Geometry check sheet. Reference: the model listing, model coordinates, mm. A direction names the side the tool comes from. Give positions to 0.01 mm unless a question says otherwise; leave off trailing zeros. Loops run counter-clockwise (first coordinate to the right, second up) from the corner with the lowest first, then second, coordinate; pieces in that order, holes last. Notation, with made-up numbers: (18, -22) - (36, -22) arc R18 cw to (36, 9) - close; hole circle Ø5 at (24, 71.25). An arc over 180 degrees is marked (long way). Use a Markdown table: item, result. Add a question column.
1. Draft check along Y on faces 1 (the flat face through (-28.228, 1.807, 9.481)), 2 (the flat face through (-57.807, 6.439, 5.009)), 3 (the flat face through (-25, 1, 0)), 4 (the flat face through (-21.915, -29.438, 11.448)). Enter one of: pulls with the +Y half, pulls with the -Y half, needs draft (parallel to the pull), parting line crosses it, or undercut.
2. Cross-section at C-C on y = 13.5. Enter the section's corners in (x, z), and give its area (3 significant figures).
3. Cross-section at B-B on x = -10. Enter the section's corners in (y, z), and give its area (3 significant figures).
4. Material ranges on L1, parallel to Y at x = -6, z = 6.5; L2, parallel to Y at x = -36, z = 8; L3, parallel to Y at x = -45, z = 7, recorded low to high.
5. Set-up check for faces 5 (the flat face through (-44.25, 18.21, 11.41)), 6 (the flat face through (-21.97, -16.81, 9.57)): record each of +Z, -Z, +X, -X, +Y, -Y from which the full face is reachable in a straight line by a thin tool's end or side.
6. Cross-section at D-D on x = -27. Enter the section's corners in (y, z).
7. Cross-section at A-A on z = 4. Enter the section's corners in (x, y).
8. Depth check by flat-ended pin: P1, Ø5, axis at x = -28, z = 5, coming from the +Y side; P2, Ø5, axis at y = -16, z = 8, coming from the +X side; P3, Ø1.9, axis at y = 14, z = 9.5, coming from the +X side. Enter the tip coordinate at first touch or a pass-through.
from build123d import *

# Parameters (mm, degrees)
F1_DEPTH    = 12.7
F3_DEPTH    = 40.64
F4_DEPTH    = 53.34
F5_T1_DEPTH = 85.1725092407
F5_T3_DEPTH = 73.3110318687
F5_T5_DEPTH = 73.3110318687
F5_T7_DEPTH = 85.1725092407
F6_SIZE     = 2.54


# Not quite as in the source:
# - a fillet or chamfer that OpenCascade refuses, or shapes differently, is made with other operations: its cross-section is extruded or revolved along the edge and cut away or added


with BuildPart() as f1:
    # F0 (on Top) → F1 (new body)
    with BuildSketch(Plane.XY):
        Polygon((0, -38.1), (0, 38.1), (-38.1, 25.4), (-52.2708785332, 12.7), (-63.5, 0), (-52.2708785332, -12.7), (-38.1, -25.4), align=None)
    extrude(amount=F1_DEPTH)

    # F2 (on face) → F3 (cut)
    with BuildSketch(Plane.YZ):
        Polygon((-14.9523484187, 6.35), (-11.2861742094, 12.7), (-18.6185226281, 12.7), align=None)
        Polygon((18.6185226281, 12.7), (11.2861742094, 12.7), (14.9523484187, 6.35), align=None)
    extrude(amount=-F3_DEPTH, mode=Mode.SUBTRACT)

    # F2 (on face) → F4 (cut)
    with BuildSketch(Plane.YZ):
        Polygon((3.6661742094, 12.7), (-3.6661742094, 12.7), (0, 6.35), align=None)
    extrude(amount=-F4_DEPTH, mode=Mode.SUBTRACT)

    # F5: chamfer of 7.62 x 12.7 on 4 edges, made by hand

    # F5_s2 → F5_t1 (cut)
    with BuildSketch(Plane.XZ.offset(-14.2269933063)):
        Polygon((-7.62, 12.7), (0, 0), (0, 12.7), align=None)
    extrude(amount=F5_T1_DEPTH, mode=Mode.SUBTRACT)

    # F5_s4 → F5_t3 (cut)
    with BuildSketch(Plane.XZ.offset(-29.179341725)):
        Polygon((-7.62, 12.7), (0, 0), (0, 12.7), align=None)
    extrude(amount=F5_T3_DEPTH, mode=Mode.SUBTRACT)

    # F5_s6 → F5_t5 (cut)
    with BuildSketch(Plane.XZ.offset(-44.1316901437)):
        Polygon((-7.62, 12.7), (0, 0), (0, 12.7), align=None)
    extrude(amount=F5_T5_DEPTH, mode=Mode.SUBTRACT)

    # F5_s8 → F5_t7 (cut)
    with BuildSketch(Plane.XZ.offset(-70.9455159344)):
        Polygon((-7.62, 12.7), (0, 0), (0, 12.7), align=None)
    extrude(amount=F5_T7_DEPTH, mode=Mode.SUBTRACT)

    # F6
    f6_edges = [f1.edges().sort_by_distance(p)[0] for p in [
        (-22.86, -30.48, 12.7),
        (-45.185439, -19.05, 12.7),
        (-57.885439, -6.35, 12.7),
        (-57.885439, 6.35, 12.7),
        (-45.185439, 19.05, 12.7),
        (-22.86, 30.48, 12.7),
    ]]
    chamfer(f6_edges, length=F6_SIZE)


solid = f1.part
Values found:
| question | item | result |
|---|---|---|
| 1 | face 1 | undercut |
| 1 | face 2 | pulls with the +Y half |
| 1 | face 3 | needs draft |
| 1 | face 4 | pulls with the -Y half |
| 2 | outline | (-51.38, 0) - (0, 0) - (-5.32, 8.87) - (-40.64, 8.87) - (-40.64, 12.7) - (-47.57, 12.7) - (-51.38, 10.16) - close |
| 2 | area | 468 mm2 |
| 3 | outline | (-34.77, 0) - (34.77, 0) - (34.77, 10.16) - (32.09, 12.7) - (18.62, 12.7) - (14.95, 6.35) - (11.29, 12.7) - (3.67, 12.7) - (0, 6.35) - (-3.67, 12.7) - (-11.29, 12.7) - (-14.95, 6.35) - (-18.62, 12.7) - (-32.09, 12.7) - (-34.77, 10.16) - close |
| 3 | area | 806 mm2 |
| 4 | L1 | y = -36.1 to -15.04, -14.87 to -0.09, 0.09 to 14.87, 15.04 to 36.1 |
| 4 | L2 | y = -26.1 to -15.9, -14 to -0.95, 0.95 to 14, 15.9 to 26.1 |
| 4 | L3 | y = -19.22 to -0.38, 0.38 to 19.22 |
| 5 | face 5 | +Z, -X, +Y |
| 5 | face 6 | +Z, +X |
| 6 | outline | (-29.1, 0) - (29.1, 0) - (29.1, 10.16) - (26.42, 12.7) - (18.62, 12.7) - (14.95, 6.35) - (11.29, 12.7) - (3.67, 12.7) - (0, 6.35) - (-3.67, 12.7) - (-11.29, 12.7) - (-14.95, 6.35) - (-18.62, 12.7) - (-26.42, 12.7) - (-29.1, 10.16) - close |
| 7 | outline | (-63.5, 0) - (-52.27, -12.7) - (-38.1, -25.4) - (-2.4, -37.3) - (-2.4, 37.3) - (-38.1, 25.4) - (-52.27, 12.7) - close |
| 8 | P1 | stops at y = 29.6 |
| 8 | P2 | stops at x = -3.3 |
| 8 | P3 | stops at x = -5.17 |
